from build123d import *

# Parameters (mm, degrees)
SKETCH1_W           = 19.5
SKETCH1_H           = 40
BOSS_EXTRUDE1_DEPTH = 2
SKETCH2_R           = 1.5
SKETCH2_W           = 5.5
SKETCH2_H           = 3
SKETCH2_W_2         = 10.5
SKETCH2_H_2         = 4.353558907
CUT_EXTRUDE1_DEPTH  = 2
SKETCH3_R           = 1.5
CUT_EXTRUDE2_DEPTH  = 2


with BuildPart() as part:
    # Sketch1 → Boss-Extrude1 (new body)
    with BuildSketch(Plane.XY):
        Rectangle(SKETCH1_W, SKETCH1_H)
    extrude(amount=BOSS_EXTRUDE1_DEPTH)

    # Sketch2 → Cut-Extrude1 (cut)
    with BuildSketch(Plane.XY.offset(2)):
        with Locations((-1.226480499, -7.435998593)):
            Circle(SKETCH2_R)
        with Locations((-5.976480499, -8.935998593)):
            Rectangle(SKETCH2_W, SKETCH2_H)
        with Locations((-3.476480499, 0.887221953)):
            Rectangle(SKETCH2_W_2, SKETCH2_H_2)
    extrude(amount=-CUT_EXTRUDE1_DEPTH, mode=Mode.SUBTRACT)

    # Sketch3 → Cut-Extrude2 (cut)
    with BuildSketch(Plane.XY.offset(2)):
        with Locations((5.75, -14)):
            Circle(SKETCH3_R)
        with Locations((5.75, 13)):
            Circle(SKETCH3_R)
    extrude(amount=-CUT_EXTRUDE2_DEPTH, mode=Mode.SUBTRACT)


solid = part.part
Geometry: final body of the model. Coordinates: model frame, mm. A direction names the side the tool comes from. Coordinates: 2 decimals unless noted, no trailing zeros. Write each loop counter-clockwise with the first axis right and the second up, starting at its lowest first coordinate (ties: lowest second). Pieces come first, ordered by that corner, then holes. Notation, with made-up numbers: (-9, 17.5) - (0, 17.5) arc R27 ccw to (0, 36.5) - close; hole circle Ø2 at (64.5, 33). An arc over 180 degrees is marked (long way). Return JSON: item names as keys, results as strings.
Item 1: Reachability of faces 4 (the face through (-3.226, -9, 1)), 5 (the face through (2, 0, 0)) from +Z, -Z, +X, -X, +Y, -Y: full face, straight path, thin tool, end or side. Return the list, or none.
Completed:
{"face 4": "+Z, -Z", "face 5": "-Z, +X, -X, +Y, -Y"}
Item 2: Line query: L1, parallel to Y at x = -7.5, z = 1.7; L2, parallel to Y at x = 5.75, z = 0.5; L3, parallel to X at y = 0.5, z = 0.5. Output: solid intervals per line, ascending.
Completed:
{"L1": "y = -20 to -10.44, -7.44 to -1.29, 3.06 to 20", "L2": "y = -20 to -15.5, -12.5 to 11.5, 14.5 to 20", "L3": "x = -9.75 to -8.73, 1.77 to 9.75"}
Item 3: Section query A-A (x = -7.25). Output: boundary loops of the cut face in (y, z).
Completed:
{"outline": "(-20, 0) - (-10.44, 0) - (-10.44, 2) - (-20, 2) - close; (-7.44, 0) - (-1.29, 0) - (-1.29, 2) - (-7.44, 2) - close; (3.06, 0) - (20, 0) - (20, 2) - (3.06, 2) - close"}
Item 4: Section query C-C (x = 1). Output: boundary loops of the cut face in (y, z).
Completed:
{"outline": "(-20, 0) - (-1.29, 0) - (-1.29, 2) - (-20, 2) - close; (3.06, 0) - (20, 0) - (20, 2) - (3.06, 2) - close"}
Item 5: Pull-direction query (X, two-part tool) for faces 1 (the face through (9.75, 0, 1)), 2 (the face through (1.774, 1, 1)), 3 (the face through (0, 20, 1)); classes: +X half, -X half, draft (parallel to the pull), parting line (faces both ways), or undercut.
Completed:
{"face 1": "+X half", "face 2": "undercut", "face 3": "draft"}
Item 6: Section query D-D (z = 0.65). Output: boundary loops of the cut face in (x, y).
Completed:
{"outline": "(-9.75, -20) - (9.75, -20) - (9.75, 20) - (-9.75, 20) - close; hole (-8.73, -10.44) - (-3.23, -10.44) - (-3.23, -7.44) - (-8.73, -7.44) - close; hole (-8.73, -1.29) - (1.77, -1.29) - (1.77, 3.06) - (-8.73, 3.06) - close; hole circle Ø3 at (-1.23, -7.44); hole circle Ø3 at (5.75, -14); hole circle Ø3 at (5.75, 13)"}
Item 7: Section query B-B (y = -14). Output: boundary loops of the cut face in (x, z).
Completed:
{"outline": "(-9.75, 0) - (4.25, 0) - (4.25, 2) - (-9.75, 2) - close; (7.25, 0) - (9.75, 0) - (9.75, 2) - (7.25, 2) - close"}
Item 8: Pin query (flat end, axial travel): pin 1 Ø10 at (x, y) = (-4, -2.5) entering from -Z; pin 2 Ø2.5 at (x, y) = (-1.23, -7.44) entering from -Z. Return the tip coordinate at first contact, or that it passes through.
Completed:
{"pin 1": "stops at z = 0", "pin 2": "passes through"}
